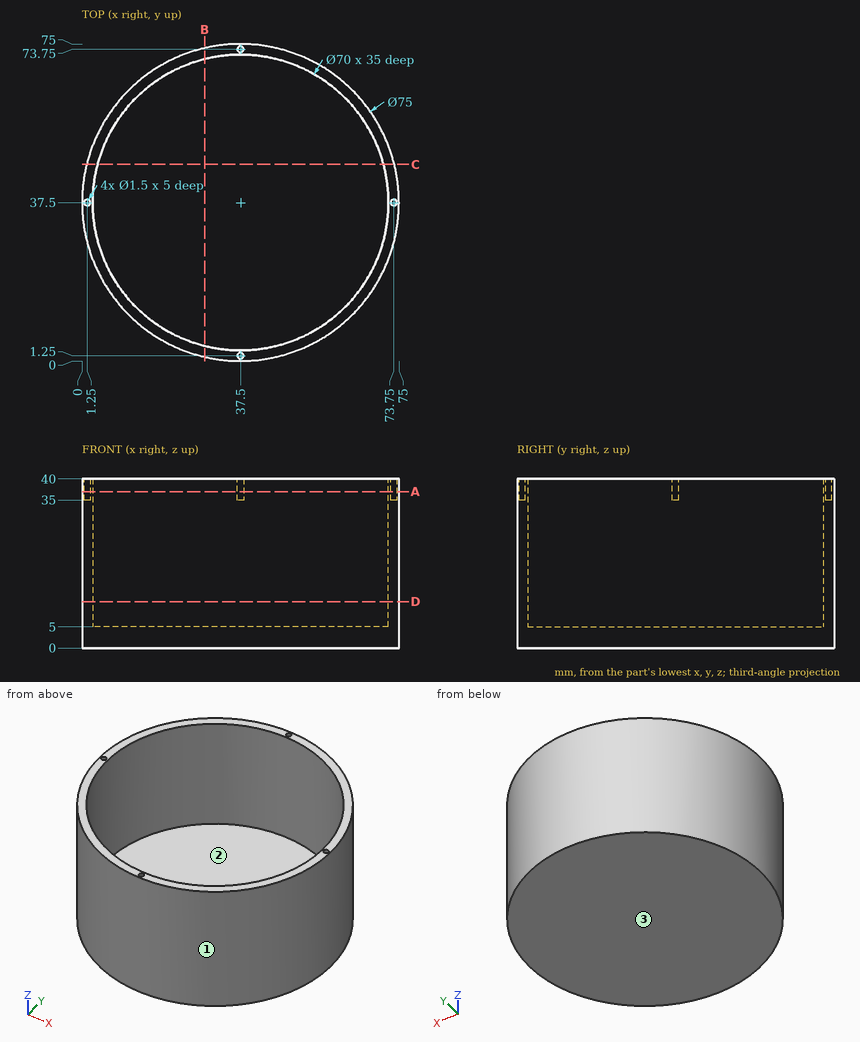
Source: three-view drawing plus pictorial views. Frame: mm from the lowest corner of the part. Give positions to 0.01 mm unless a question says otherwise; leave off trailing zeros. Order: outer loops, then holes, each group sorted by start corner. A loop starts at its lowest first (then second) coordinate and runs counter-clockwise, first axis right, second up. Notation, with made-up numbers: (-36.5, -36.75) -> (-2.5, -36.75) arc R12 cw to (-2.5, -21.75) -> close; hole circle Ø8 at (41, 61). An arc over 180 degrees is marked (long way). Use a Markdown table: item, result.
Q1. Section D-D (z = 11). Return the cut outline in (x, y), and give its area (3 significant figures).
A:
| item | result |
|---|---|
| outline | circle Ø75 at (37.5, 37.5); hole circle Ø70 at (37.5, 37.5) |
| area | 569 mm^2 |
Q2. Section B-B (x = 29). Return the cut outline in (y, z), and give its area (3 significant figures).
A:
| item | result |
|---|---|
| outline | (0.98, 0) -> (74.02, 0) -> (74.02, 40) -> (71.45, 40) -> (71.45, 5) -> (3.55, 5) -> (3.55, 40) -> (0.98, 40) -> close |
| area | 545 mm^2 |
Q3. Section C-C (y = 46.5). Return the cut outline in (x, z), and give its area (3 significant figures).
A:
| item | result |
|---|---|
| outline | (1.1, 0) -> (73.9, 0) -> (73.9, 40) -> (71.32, 40) -> (71.32, 5) -> (3.68, 5) -> (3.68, 40) -> (1.1, 40) -> close |
| area | 545 mm^2 |
Q4. Pull-direction query (X, two-part tool) for the marked faces 1, 2 and 3; classes: +X half, -X half, draft (parallel to the pull), parting line (faces both ways), or undercut.
A:
| item | result |
|---|---|
| face 1 | parting line |
| face 2 | undercut |
| face 3 | draft |
Q5. Material intervals for line 1 (Y direction, x = 37.5, z = 36.15); line 2 (X direction, y = 37, z = 17); line 3 (X direction, y = 37, z = 37), sorted ascending. Write a range as [from, to].
A:
| item | result |
|---|---|
| line 1 | [0, 0.5], [2, 2.5], [72.5, 73], [74.5, 75] |
| line 2 | [0, 2.5], [72.5, 75] |
| line 3 | [0, 0.69], [1.81, 2.5], [72.5, 73.19], [74.31, 75] |
Q6. First-contact query: P1, Ø1.5, axis at x = 40.5, z = 31, coming from the +Y side; P2, Ø1.5, axis at x = 44.5, z = 30, coming from the +Y side; P3, Ø4, axis at y = 22, z = 33, coming from the +X side. Flat tips, straight axial feed; report the tip coordinate or a pass-through.
A:
| item | result |
|---|---|
| P1 | y = 74.93 |
| P2 | y = 74.48 |
| P3 | x = 72.49 |
Q7. Section A-A (z = 37). Return the cut outline in (x, y).
A:
| item | result |
|---|---|
| outline | circle Ø75 at (37.5, 37.5); hole circle Ø1.5 at (1.25, 37.5); hole circle Ø70 at (37.5, 37.5); hole circle Ø1.5 at (37.5, 1.25); hole circle Ø1.5 at (37.5, 73.75); hole circle Ø1.5 at (73.75, 37.5) |
